CAD build for the part. Positions are in the model's coordinates, mm. Face numbers are marked on the shaded views. A direction names the side the tool comes from. Give positions to 0.01 mm unless a question says otherwise; leave off trailing zeros. Loops run counter-clockwise (first coordinate to the right, second up) from the corner with the lowest first, then second, coordinate; pieces in that order, holes last.
Item 1: Saw through at A-A on x = 4. Give the cut face in (y, z).
Item 2: Probe probe 1 along Z at (x, y) = (2.25, 0); probe 2 along Z at (x, y) = (0.75, -0.45); probe 3 along Z at (x, y) = (1.5, 0). List the from-to ranges inside material, lowest first.
Item 3: Which spindle directions (+Z, -Z, +X, -X, +Y, -Y) get a long thin tool onto all of the face, cutting with end or side? Do the marked faces 1 and 2. Say none if no direction does.
Item 4: Drop flat-ended pins along their axis: P1, Ø3, axis at y = 2, z = -0.5, coming from the -X side; P2, Ø1, axis at x = 1, z = 0.5, coming from the +Y side; P3, Ø1, axis at x = 4.5, z = -1, coming from the -Y side; P4, Ø2, axis at x = 4.5, z = -1, coming from the -Y side. Give the stop position or say it passes through.
Item 5: Mould opens along Y. For the marked faces 3, 4, 5 and 6 say: released by +Y, released by -Y, zero draft, split by the parting line, or undercut.
from build123d import *

# Parameters (mm, degrees)
FILLET1_R     = 0.8
SKETCH3_W     = 0.74
SKETCH3_H     = 3
SKETCH4_W     = 0.74
SKETCH4_H     = 0.995702004
RECPAT_COUNT  = 2
RECPAT_ANGLE  = 90
CHANFRO1_SIZE = 0.25


with BuildPart() as part:
    # BodySke → Base-Revolve (revolve)
    with BuildSketch(Plane.XY):
        Polygon((0, 0), (0, 2.75), (0.4, 2.75), (1.65, 1.5), (6, 1.5), (6, 0), align=None)
    revolve(axis=Axis((-6.35, 0, 0), (1, 0, 0)))

    # Fillet1
    fillet1_edges = [part.edges().sort_by_distance(p)[0] for p in [
        (1.65, -1.5, 0),
    ]]
    fillet(fillet1_edges, radius=FILLET1_R)

    # Sketch3 → Recess section 0
    with BuildSketch(Plane.ZY):
        Rectangle(SKETCH3_W, SKETCH3_H)
    # Sketch4 → Recess section 1
    with BuildSketch(Plane.ZY.offset(-2.01)):
        Rectangle(SKETCH4_W, SKETCH4_H)
    recess = loft(mode=Mode.SUBTRACT)

    # RecPat: Recess ×2 about axis
    recpat_axis = Axis((0, 0, 0), (1, 0, 0))
    for i in range(1, RECPAT_COUNT):
        add(recess.rotate(recpat_axis, i * RECPAT_ANGLE / (RECPAT_COUNT - 1)), mode=Mode.SUBTRACT)

    # RecCorSke → RecessCore (revolve, cut)
    with BuildSketch(Plane.XY):
        Polygon((0, 0), (0, 0.696552892), (2.01, 0.556), (2.190655351, 0), align=None)
    revolve(axis=Axis((-3.175, 0, 0), (1, 0, 0)), mode=Mode.SUBTRACT)

    # Chanfro1
    chanfro1_edges = [part.edges().sort_by_distance(p)[0] for p in [
        (6, -1.5, 0),
    ]]
    chamfer(chanfro1_edges, length=CHANFRO1_SIZE)


solid = part.part
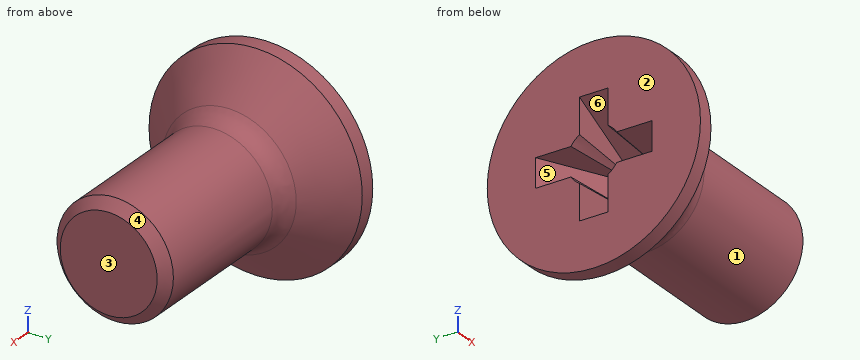
Results below:
1. outline: circle Ø3 at (0, 0)
2. probe 1: z = -1.5 to 1.5
2. probe 2: z = -2.36 to -0.46, 0.46 to 2.36
2. probe 3: z = -1.66 to -0.75, 0.75 to 1.66
3. face 1: +X
3. face 2: +Z, -Z, -X, +Y, -Y
4. P1: stops at x = 0
4. P2: stops at y = 2.61
4. P3: stops at y = -1.41
4. P4: stops at y = -1.5
5. face 3: zero draft
5. face 4: split by the parting line
5. face 5: undercut
5. face 6: undercut
